from build123d import *

# Parameters (mm, degrees)
BOSS_EXTRUDE1_DEPTH        = 1.5
SKETCH2_W                  = 2.7
SKETCH2_H                  = 5.4
BOSS_EXTRUDE2_DEPTH        = 2
CHAMFER1_SIZE              = 0.2
SKETCH3_W                  = 1.410498469
SKETCH3_H                  = 0.5
BOSS_EXTRUDE3_DEPTH        = 0.7
CHAMFER2_SIZE              = 1
LPATTERN2_COUNT            = 4
LPATTERN2_PITCH            = 1.25
CHAMFER2_OF_LPATTERN2_SIZE = 1
MIRROR1_START              = -9.5
MIRROR1_DEPTH              = 5.4
MIRROR1_START_2            = -9
MIRROR1_2_DEPTH            = 0.5
MIRROR1_START_3            = -7.75
MIRROR1_3_DEPTH            = 0.5
MIRROR1_START_4            = -6.5
MIRROR1_4_DEPTH            = 0.5
MIRROR1_START_5            = -5.25
MIRROR1_5_DEPTH            = 0.5
MIRROR1_START_6            = -0.565685425
MIRROR1_6_OUTLINE_W        = 4.6
MIRROR1_6_OUTLINE_H        = 5.050966799
MIRROR1_6_DEPTH            = 1.565685425
MIRROR1_START_7            = -5
MIRROR1_7_OUTLINE_W        = 4.6
MIRROR1_7_OUTLINE_H        = 1.949033201
MIRROR1_7_DEPTH            = 4.434314575
SKETCH5_W                  = 2.5
SKETCH5_H                  = 10
BOSS_EXTRUDE4_DEPTH        = 2.5
SKETCH6_W                  = 0.5
SKETCH6_H                  = 0.5
BOSS_EXTRUDE5_DEPTH        = 7
LPATTERN3_COUNT            = 4
LPATTERN3_PITCH            = 2.5


with BuildPart() as part:
    # Sketch1 → Boss-Extrude1 (new body)
    with BuildSketch(Plane(origin=(0, 0, 0), x_dir=(1, 0, 0), z_dir=(0, 1, 0))):
        with BuildLine():
            Line((-19.2, 0), (0, 0))
            Line((0, 0), (0, 13.6))
            Line((0, 13.6), (-12.7, 13.6))
            ThreePointArc((-12.7, 13.6), (-14.2, 12.1), (-15.7, 13.6))
            Line((-15.7, 13.6), (-19.2, 13.6))
            Line((-19.2, 13.6), (-19.2, 0))
        make_face()
    extrude(amount=BOSS_EXTRUDE1_DEPTH)

    # Sketch2 → Boss-Extrude2 (add)
    with BuildSketch(Plane(origin=(0, 1.5, 0), x_dir=(1, 0, 0), z_dir=(0, 1, 0))):
        with Locations((-10.95, 6.8)):
            Rectangle(SKETCH2_W, SKETCH2_H)
    extrude(amount=BOSS_EXTRUDE2_DEPTH)

    # Chamfer1
    chamfer1_edges = [part.edges().sort_by_distance(p)[0] for p in [
        (-12.3, 3.5, -6.8),
        (-10.95, 3.5, -4.1),
        (-10.95, 3.5, -9.5),
    ]]
    chamfer(chamfer1_edges, length=CHAMFER1_SIZE)

    # Sketch3 → Boss-Extrude3 (add)
    with BuildSketch(Plane(origin=(0, 1.5, 0), x_dir=(1, 0, 0), z_dir=(0, 1, 0))):
        with Locations((-13.005249235, 8.75)):
            Rectangle(SKETCH3_W, SKETCH3_H)
    boss_extrude3 = extrude(amount=BOSS_EXTRUDE3_DEPTH)

    # Chamfer2
    # the kernel refuses this chamfer: 1 mm, written as the material it takes off along each edge
    with BuildSketch(Plane(origin=(-13.710498469, 2.2, -11.571682988), x_dir=(1, 0, 0), z_dir=(0, 0, 1))) as chamfer2_piece_1_section:
        Polygon((CHAMFER2_SIZE, 0), (0, -CHAMFER2_SIZE), (0, 0), align=None)
    chamfer2_piece_1 = extrude(amount=5.643365976, mode=Mode.PRIVATE)
    chamfer2_piece_1 = split(chamfer2_piece_1, bisect_by=Plane(origin=(-13.710498469, 1.5, -11.571682988), z_dir=(0, 1, 0)), keep=Keep.TOP, mode=Mode.PRIVATE)
    add(chamfer2_piece_1, mode=Mode.SUBTRACT)

    # LPattern2: Boss-Extrude3 ×4
    with Locations(*[(0, 0, i * LPATTERN2_PITCH) for i in range(1, LPATTERN2_COUNT)]):
        add(boss_extrude3)

    # Chamfer2 of LPattern2
    # the kernel refuses this chamfer: 1 mm, written as the material it takes off along each edge
    with BuildSketch(Plane(origin=(-13.710498469, 2.2, -10.321682988), x_dir=(1, 0, 0), z_dir=(0, 0, 1))) as chamfer2_of_lpattern2_piece_1_section:
        Polygon((CHAMFER2_OF_LPATTERN2_SIZE, 0), (0, -CHAMFER2_OF_LPATTERN2_SIZE), (0, 0), align=None)
    chamfer2_of_lpattern2_piece_1 = extrude(amount=5.643365976, mode=Mode.PRIVATE)
    chamfer2_of_lpattern2_piece_1 = split(chamfer2_of_lpattern2_piece_1, bisect_by=Plane(origin=(-13.710498469, 1.5, -10.321682988), z_dir=(0, 1, 0)), keep=Keep.TOP, mode=Mode.PRIVATE)
    add(chamfer2_of_lpattern2_piece_1, mode=Mode.SUBTRACT)
    with BuildSketch(Plane(origin=(-13.710498469, 2.2, -9.071682988), x_dir=(1, 0, 0), z_dir=(0, 0, 1))) as chamfer2_of_lpattern2_piece_2_section:
        Polygon((CHAMFER2_OF_LPATTERN2_SIZE, 0), (0, -CHAMFER2_OF_LPATTERN2_SIZE), (0, 0), align=None)
    chamfer2_of_lpattern2_piece_2 = extrude(amount=5.643365976, mode=Mode.PRIVATE)
    chamfer2_of_lpattern2_piece_2 = split(chamfer2_of_lpattern2_piece_2, bisect_by=Plane(origin=(-13.710498469, 1.5, -9.071682988), z_dir=(0, 1, 0)), keep=Keep.TOP, mode=Mode.PRIVATE)
    add(chamfer2_of_lpattern2_piece_2, mode=Mode.SUBTRACT)
    with BuildSketch(Plane(origin=(-13.710498469, 2.2, -7.821682988), x_dir=(1, 0, 0), z_dir=(0, 0, 1))) as chamfer2_of_lpattern2_piece_3_section:
        Polygon((CHAMFER2_OF_LPATTERN2_SIZE, 0), (0, -CHAMFER2_OF_LPATTERN2_SIZE), (0, 0), align=None)
    chamfer2_of_lpattern2_piece_3 = extrude(amount=5.643365976, mode=Mode.PRIVATE)
    chamfer2_of_lpattern2_piece_3 = split(chamfer2_of_lpattern2_piece_3, bisect_by=Plane(origin=(-13.710498469, 1.5, -7.821682988), z_dir=(0, 1, 0)), keep=Keep.TOP, mode=Mode.PRIVATE)
    add(chamfer2_of_lpattern2_piece_3, mode=Mode.SUBTRACT)

    # Mirror1: read off the stored shape, not the designer's step
    # Mirror1 outline → Mirror1 (add)
    with BuildSketch(Plane.XY.offset(MIRROR1_START)):
        Polygon((-6.9, 3.3), (-7.1, 3.5), (-9.6, 3.5), (-9.6, 1.5), (-6.9, 1.5), align=None)
    extrude(amount=MIRROR1_DEPTH)

    # Mirror1 2 outline → Mirror1 2 (add)
    with BuildSketch(Plane.XY.offset(MIRROR1_START_2)):
        Polygon((-6.489501531, 2.2), (-6.9, 2.2), (-6.9, 1.5), (-5.789501531, 1.5), align=None)
    extrude(amount=MIRROR1_2_DEPTH)

    # Mirror1 3 outline → Mirror1 3 (add)
    with BuildSketch(Plane.XY.offset(MIRROR1_START_3)):
        Polygon((-6.489501531, 2.2), (-6.9, 2.2), (-6.9, 1.5), (-5.789501531, 1.5), align=None)
    extrude(amount=MIRROR1_3_DEPTH)

    # Mirror1 4 outline → Mirror1 4 (add)
    with BuildSketch(Plane.XY.offset(MIRROR1_START_4)):
        Polygon((-6.489501531, 2.2), (-6.9, 2.2), (-6.9, 1.5), (-5.789501531, 1.5), align=None)
    extrude(amount=MIRROR1_4_DEPTH)

    # Mirror1 5 outline → Mirror1 5 (add)
    with BuildSketch(Plane.XY.offset(MIRROR1_START_5)):
        Polygon((-6.489501531, 2.2), (-6.9, 2.2), (-6.9, 1.5), (-5.789501531, 1.5), align=None)
    extrude(amount=MIRROR1_5_DEPTH)

    # Mirror1 6 outline → Mirror1 6 (cut)
    with BuildSketch(Plane(origin=(0, 0, 0), x_dir=(1, 0, 0), z_dir=(0, 0.707106781186545, 0.70710678118655)).offset(MIRROR1_START_6)):
        with Locations((-7.3, 6.5254834)):
            Rectangle(MIRROR1_6_OUTLINE_W, MIRROR1_6_OUTLINE_H)
    extrude(amount=MIRROR1_6_DEPTH, mode=Mode.SUBTRACT)

    # Mirror1 7 outline → Mirror1 7 (cut)
    with BuildSketch(Plane(origin=(0, 0, 0), x_dir=(1, 0, 0), z_dir=(0, 0.707106781186545, 0.70710678118655)).offset(MIRROR1_START_7)):
        with Locations((-7.3, 10.0254834)):
            Rectangle(MIRROR1_7_OUTLINE_W, MIRROR1_7_OUTLINE_H)
    extrude(amount=MIRROR1_7_DEPTH, mode=Mode.SUBTRACT)

    # Sketch5 → Boss-Extrude4 (add)
    with BuildSketch(Plane.XZ):
        with Locations((-15.85, -6.8)):
            Rectangle(SKETCH5_W, SKETCH5_H)
        with Locations((-3.35, -6.8)):
            Rectangle(SKETCH5_W, SKETCH5_H)
    extrude(amount=BOSS_EXTRUDE4_DEPTH)

    # Sketch6 → Boss-Extrude5 (add)
    with BuildSketch(Plane.XZ.offset(2.5)):
        with Locations((-15.85, -3.05)):
            Rectangle(SKETCH6_W, SKETCH6_H)
        with Locations((-3.35, -3.05)):
            Rectangle(SKETCH6_W, SKETCH6_H)
    boss_extrude5 = extrude(amount=BOSS_EXTRUDE5_DEPTH)

    # LPattern3: Boss-Extrude5 ×4
    with Locations(*[(0, 0, -i * LPATTERN3_PITCH) for i in range(1, LPATTERN3_COUNT)]):
        add(boss_extrude5)


solid = part.part
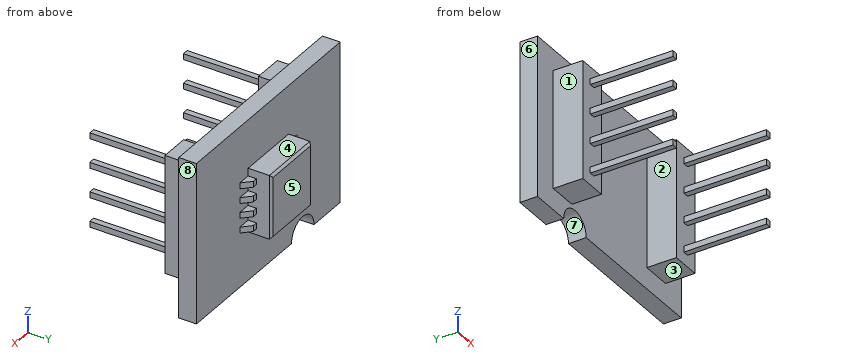
Model file for the job. Use its own axes, mm. Face numbers are marked on the shaded views. A direction names the side the tool comes from. Give positions to 0.01 mm unless a question says otherwise; leave off trailing zeros. Write each loop counter-clockwise with the first axis right and the second up, starting at its lowest first coordinate (ties: lowest second). Pieces come first, ordered by that corner, then holes. Notation, with made-up numbers: M -40,50.5 L -25,50.5 A24 ccw -25,74.5 Z; hole C -1.75,70 d1. An arc over 180 degrees is marked long. One line per item, written item: value. Start each with the question number.
Q1. Saw through at B-B, the plane y = -1. Write the cut outline in (x, z), plus the area to 3 significant figures.
Q2. Saw through at A-A, the plane y = -7.5. State how many separate pieces and enclosed holes the cut face has, plus the area to 3 significant figures.
Q3. Drop flat-ended pins along their axis: pin 1 Ø1.5 at (x, z) = (-8.5, -8.5) entering from -Y; pin 2 Ø4 at (y, z) = (-4, -9.5) entering from +X; pin 3 Ø6 at (y, z) = (-6.5, -8) entering from -X. Give the stop position or say it passes through.
Q4. Probe probe 1 along X at (y, z) = (-0.25, -8); probe 2 along Y at (x, z) = (-5, -4.5); probe 3 along Z at (x, y) = (-14.75, -0.5). List the from-to ranges inside material, lowest first. Write a range as [from, to].
Q5. Two-plate mould, pull along X, no slides. Class the marked faces 6, 7 and 8: +X half, -X half, draft (parallel to the pull), parting line (faces both ways), or undercut.
Q6. 3-axis set-ups, long thin cutter, end or side, ignore diameter. For the marked faces 1, 2, 3, 4 and 5: which of +Z, -Z, +X, -X, +Y, -Y reach the whole face in a straight line?
Q7. Saw through at C-C, the plane x = -14.2. Write the cut outline in (y, z), plus the area to 4 significant figures.
Output values:
1. outline: M -17.1,-11.8 L -14.6,-11.8 L -14.6,-1.8 L -17.1,-1.8 Z; M -4.6,-11.8 L -2.1,-11.8 L -2.1,-1.8 L -4.6,-1.8 Z
1. area: 50.0 mm²
2. separate pieces: 8
2. enclosed holes: 0
2. area: 2.00 mm²
3. pin 1: stops at y = 0
3. pin 2: stops at x = -2.1
3. pin 3: stops at x = -16.1
4. probe 1: x = [-17.1, -14.6], [-4.6, -2.1]
4. probe 2: y = [0, 1.5]
4. probe 3: z = [-11.8, -1.8]
5. face 6: -X half
5. face 7: undercut
5. face 8: +X half
6. face 1: +Z, -Z, -X, -Y
6. face 2: +Z, -Z, -Y
6. face 3: -Z, +X, -X, -Y
6. face 4: +Z, +X, -X, +Y
6. face 5: +Z, -Z, +X, -X, +Y
7. outline: M 0,-12.1 L 1.5,-12.1 L 1.5,0 L 0,0 Z
7. area: 18.15 mm²
